Check sheet for the modelled part. Datum: model origin and axes. Units: mm. Face numbers are marked on the shaded views. A direction names the side the tool comes from. Round coordinates to 2 decimals unless told otherwise and drop trailing zeros. Write each loop counter-clockwise with the first axis right and the second up, starting at its lowest first coordinate (ties: lowest second). Pieces come first, ordered by that corner, then holes. Notation, with made-up numbers: (79, -33.75) - (88, -33.75) arc R15 cw to (88, -6.75) - close; hole circle Ø1 at (87, 8). An arc over 180 degrees is marked (long way). Answer as a JSON object with one key per item and string values. Group by question number.
Item 1: Release check for a two-part mould opening along Y. For the marked faces 1, 2 and 3 record: pulls with the +Y half, pulls with the -Y half, needs draft (parallel to the pull), parting line crosses it, or undercut.
Item 2: Sectioned sample at A-A on x = 0. Record the boundary of the cut face in (y, z), plus the area to 3 significant figures.
Item 3: Sectioned sample at D-D on x = -5.5. Record the boundary of the cut face in (y, z).
Item 4: Gauge pin test, flat ends, axial feed: P1, Ø1.2, axis at x = -6, z = 21.5, coming from the -Y side; P2, Ø3, axis at x = -3.5, z = 24.5, coming from the +Y side; P3, Ø0.9, axis at y = 1, z = 7.5, coming from the +X side. Record the tip position at first contact, or that the pin passes through.
Item 5: Sectioned sample at C-C on y = -0.75. Record the boundary of the cut face in (x, z).
Item 6: Set-up check for the marked faces 4, 5 and 6: record each of +Z, -Z, +X, -X, +Y, -Y from which the full face is reachable in a straight line by a thin tool's end or side.
Item 7: Sectioned sample at B-B on z = 22. Record the boundary of the cut face in (x, y).
Item 8: Thickness scan on line 1 (Y direction, x = 0, z = 8.5); line 2 (X direction, y = 0, z = 13.5); line 3 (Z direction, x = -3.75, y = 1). Record the ranges inside material, lowest first.
Solid Edge part; units mm, degrees
sketch "Sketch1" plane through (0, 0, 0) normal (0, 0, 1) x (1, 0, 0)
  circle A0 centre (0, 0) radius 7.5
extrude "Protrusion1" add sketch "Sketch1" along normal blind 30
sketch "Sketch2" plane through (0, 0, 30) normal (0, 0, 1) x (1, 0, 0)
  circle A0 centre (0, 0) radius 2.1
extrude "ExtrudedCutout_1" cut sketch "Sketch2" against normal blind 15
sketch "Sketch3" plane through (0, 0, 0) normal (0, 0, -1) x (1, 0, 0)
  line L0 (-2.0799, -1.5601) -> (-2.0799, 1.5601)
  arc A0 (-2.0799, 1.5601) -> (-2.0799, -1.5601) centre (0, 0) cw
extrude "Cutout1" cut sketch "Sketch3" against normal up to vertex (15 mm away)
sketch "Sketch4" plane through (-7.5, 0, 15) normal (-1, 0, 0) x (0, 0, -1)
  line L0 (5.4123, 2.75) -> (3.8246, 0)
  line L1 (3.8246, 0) -> (5.4123, -2.75)
  line L2 (5.4123, -2.75) -> (8.5877, -2.75)
  line L3 (8.5877, -2.75) -> (10.1754, 0)
  line L4 (10.1754, 0) -> (8.5877, 2.75)
  line L5 (8.5877, 2.75) -> (5.4123, 2.75)
  line L6 (-8.5877, 2.75) -> (-10.1754, 0)
  line L7 (-10.1754, 0) -> (-8.5877, -2.75)
  line L8 (-8.5877, -2.75) -> (-5.4123, -2.75)
  line L9 (-5.4123, -2.75) -> (-3.8246, 0)
  line L10 (-3.8246, 0) -> (-5.4123, 2.75)
  line L11 (-5.4123, 2.75) -> (-8.5877, 2.75)
extrude "ExtrudedCutout_3" cut sketch "Sketch4" against normal blind 3
sketch "Sketch5" plane through (-7.5, 0, 15) normal (-1, 0, 0) x (0, 0, -1)
  circle A0 centre (-7, 0) radius 1.35
  circle A1 centre (7, 0) radius 1.35
extrude "Cutout2" cut sketch "Sketch5" against normal up to next
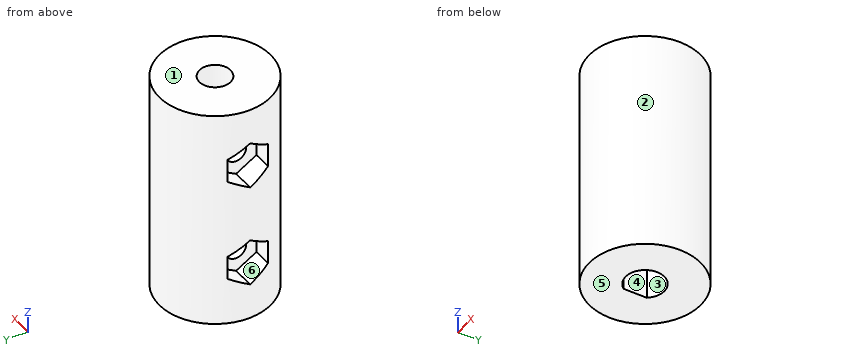
Completed:
{
 "1": {"face 1": "needs draft", "face 2": "parting line crosses it", "face 3": "undercut"},
 "2": {"outline": "(-7.5, 0) - (-2.6, 0) - (-2.6, 15) - (-2.1, 15) - (-2.1, 30) - (-7.5, 30) - close; (2.1, 15) - (2.6, 15) - (2.6, 0) - (7.5, 0) - (7.5, 30) - (2.1, 30) - close", "area": "309 mm²"},
 "3": {"outline": "(-5.1, 0) - (5.1, 0) - (5.1, 30) - (-5.1, 30) - close; hole (-2.75, 6.41) - (0, 4.82) - (2.75, 6.41) - (2.75, 9.59) - (0, 11.18) - (-2.75, 9.59) - close; hole (-2.75, 20.41) - (0, 18.82) - (2.75, 20.41) - (2.75, 23.59) - (0, 25.18) - (-2.75, 23.59) - close"},
 "4": {"P1": "y = -5.2", "P2": "y = 7.23", "P3": "x = 7.48"},
 "5": {"outline": "(-7.46, 0) - (-2.08, 0) - (-2.08, 6.88) - (-4.5, 6.88) - (-4.5, 5.26) - (-7.46, 5.26) - close; (-7.46, 10.74) - (-4.5, 10.74) - (-4.5, 9.12) - (-2.08, 9.12) - (-2.08, 15) - (-1.96, 15) - (-1.96, 20.88) - (-4.5, 20.88) - (-4.5, 19.26) - (-7.46, 19.26) - close; (-7.46, 24.74) - (-4.5, 24.74) - (-4.5, 23.12) - (-1.96, 23.12) - (-1.96, 30) - (-7.46, 30) - close; (1.96, 15) - (2.49, 15) - (2.49, 0) - (7.46, 0) - (7.46, 30) - (1.96, 30) - close"},
 "6": {"face 4": "-Z", "face 5": "-Z, +X, -X, +Y, -Y", "face 6": "-X"},
 "7": {"outline": "(-6.98, -2.75) arc R7.5 ccw (long way) to (-6.98, 2.75) - (-4.5, 2.75) - (-4.5, 1.35) - (-1.61, 1.35) arc R2.1 cw (long way) to (-1.61, -1.35) - (-4.5, -1.35) - (-4.5, -2.75) - close"},
 "8": {"line 1": "-7.5 to -2.6, 2.6 to 7.5", "line 2": "-7.5 to -2.08, 2.6 to 7.5", "line 3": "0 to 7.09, 8.91 to 21.09, 22.91 to 30"}
}
